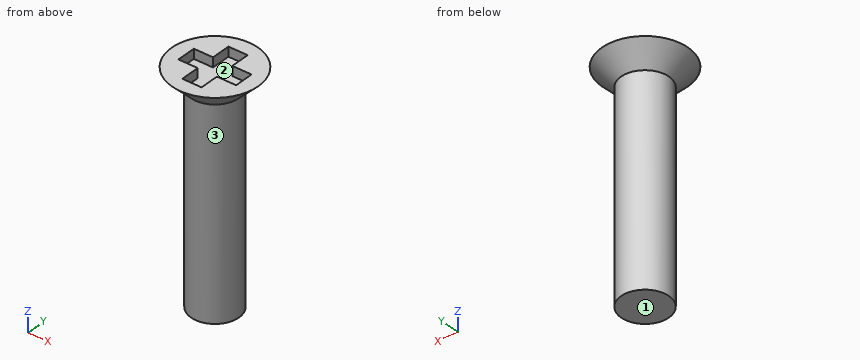
```python
from build123d import *

# Parameters (mm, degrees)
F0_R      = 3.175
F1_DEPTH  = 27.305
F1_FACE_R = 3.175
F2_DEPTH  = 2.54
F2_TAPER  = -45
F3_W      = 2.54
F3_H      = 2.54
F4_DEPTH  = 1.27


with BuildPart() as f1:
    # F0 (on Top) → F1 (new body)
    with BuildSketch(Plane.XY):
        Circle(F0_R)
    extrude(amount=F1_DEPTH)

    # F1_face (on face) → F2 (join)
    with BuildSketch(Plane.XY.offset(27.305)):
        Circle(F1_FACE_R)
    extrude(amount=F2_DEPTH, taper=F2_TAPER)

    # F3 (on face) → F4 (cut)
    with BuildSketch(Plane.XY.offset(29.845)):
        with Locations((0, 2.54)):
            Rectangle(F3_W, F3_H)
        with Locations((-2.54, 0)):
            Rectangle(F3_W, F3_H)
        Rectangle(F3_W, F3_H)
        with Locations((2.54, 0)):
            Rectangle(F3_W, F3_H)
        with Locations((0, -2.54)):
            Rectangle(F3_W, F3_H)
    extrude(amount=-F4_DEPTH, mode=Mode.SUBTRACT)


solid = f1.part
```
For this review, take the finished solid that the model builds, in its own axes (mm). Face numbers are marked on the shaded views. Give positions to 0.01 mm unless a question says otherwise; leave off trailing zeros. Write each loop counter-clockwise with the first axis right and the second up, starting at its lowest first coordinate (ties: lowest second). Pieces come first, ordered by that corner, then holes. Notation, with made-up numbers: M -35.5,13 L 4.5,13 A13 cw 4.5,34 Z; hole C 45,37 d9. An arc over 180 degrees is marked long. One line per item, written item: value.
1) For line 1 (Z direction, x = 0, y = -2.25) (3 decimals); line 2 (Y direction, x = 1.5, z = 8.5); line 3 (Y direction, x = 1, z = 22.25), list the stretches that pass through material, from the lowest coordinate up. Write a range as from..to.
Results are:
line 1: z = 0..28.575
line 2: y = -2.8..2.8
line 3: y = -3.01..3.01
2) Take a section at A-A, the plane x = 0. Write out the cut boundary in (y, z) (3 decimals).
Results are:
outline: M -5.715,29.845 L -3.175,27.305 L -3.175,0 L 3.175,0 L 3.175,27.305 L 5.715,29.845 L 3.81,29.845 L 3.81,28.575 L -3.81,28.575 L -3.81,29.845 Z
3) The part is to be moulded in two halves that separate along Y. For the marked faces 1, 2 and 3, say which applies: +Y half, -Y half, draft (parallel to the pull), parting line (faces both ways), or undercut.
Results are:
face 1: draft
face 2: undercut
face 3: parting line
4) Take a section at B-B, the plane z = 11.5. Write out the cut boundary in (x, y) (3 decimals), then the cut area to 3 significant figures.
Results are:
outline: C 0,0 d6.35
area: 31.7 mm²
5) For P1, Ø0.6, axis at y = -2.5, z = 29, coming from the +X side; P2, Ø4, axis at x = 1.5, z = 7.5, coming from the +Y side (3 decimals); P3, Ø1.4, axis at x = 3, z = 29.5, coming from the +Y side, all flat-tipped, find the tip position at first contact; note any pin that passes through.
Results are:
P1: stops at x = 4.56
P2: stops at y = 3.175
P3: stops at y = 5.19
